Geometry: final body of the model. Coordinates: model frame, mm. A direction names the side the tool comes from. Coordinates: 2 decimals unless noted, no trailing zeros. Write each loop counter-clockwise with the first axis right and the second up, starting at its lowest first coordinate (ties: lowest second). Pieces come first, ordered by that corner, then holes. Notation, with made-up numbers: M 34.5,27.5 L 38.5,27.5 A23 ccw 38.5,49.5 Z; hole C 35.5,89 d7. An arc over 180 degrees is marked long. Write item = value, one per line. Start each with the question number.
Item 1: Reachability of faces 1 (the flat face through (-2.5, -25, 5)), 2 (the flat face through (15, 21, 5)), 3 (the flat face through (-20, 11.5, 7)), 4 (the flat face through (-9, 8, 1)), 5 (the flat face through (-24.2, -15.4, 3.9)) from +Z, -Z, +X, -X, +Y, -Y: full face, straight path, thin tool, end or side. Return the list, or none.
Item 2: Section A-A on y = 21.5. Output: boundary loops of the cut face in (x, z), plus the area to 3 significant figures.
Item 3: Ray query, L1, parallel to X at y = -5, z = 0.75; L2, parallel to Y at x = 15.5, z = 2.75; L3, parallel to Y at x = -16, z = 6. Return the intervals inside material, ascending. Write a range as [from, to].
Item 4: Section C-C on y = -21.5. Output: boundary loops of the cut face in (x, z).
Item 5: Section D-D on y = -10. Output: boundary loops of the cut face in (x, z).
Item 6: First-contact query: pin 1 Ø0.6 at (y, z) = (-17, 0.5) entering from +X; pin 2 Ø6 at (x, y) = (-5.5, -0.5) entering from +Z; pin 3 Ø4 at (y, z) = (1, 4.5) entering from -X; pin 4 Ø10 at (x, y) = (13.5, -2.5) entering from -Z. Flat tips, straight axial feed; report the tip coordinate or a pass-through.
Item 7: Pull-direction query (Y, two-part tool) for faces 6 (the flat face through (0, -6, 0)), 7 (the flat face through (-14, 11, 1)); classes: +Y half, -Y half, draft (parallel to the pull), parting line (faces both ways), or undercut.
Item 8: Section B-B on x = 10. Output: boundary loops of the cut face in (y, z).
from build123d import *

# Parameters (mm, degrees)
SKETCH1_W                                  = 41
SKETCH1_H                                  = 51
BOSS_EXTRUDE1_DEPTH                        = 8
SHELL1_T                                   = -2
CUT_EXTRUDE1_DEPTH                         = 34.264094757
SKETCH3_W                                  = 10
SKETCH3_H                                  = 5
CUT_EXTRUDE2_DEPTH                         = 7
SKETCH4_W                                  = 2
SKETCH4_H                                  = 14
CUT_EXTRUDE3_DEPTH                         = 7
SKETCH5_W                                  = 3.5
SKETCH5_H                                  = 22
CUT_EXTRUDE4_DEPTH                         = 7
SKETCH6_R                                  = 1.75
BOSS_EXTRUDE2_DEPTH                        = 8
MIRROR1_AT_THE_SECOND_PLANE_COPY_1_SKETC_R = 1.75
MIRROR1_AT_THE_SECOND_PLANE_COPY_1_DEPTH   = 8
SKETCH7_W                                  = 9.5
SKETCH7_H                                  = 5.5
BOSS_EXTRUDE3_DEPTH                        = 3
CHAMFER1_SIZE                              = 3


with BuildPart() as part:
    # Sketch1 → Boss-Extrude1 (new body)
    with BuildSketch(Plane.XY):
        Rectangle(SKETCH1_W, SKETCH1_H)
    extrude(amount=BOSS_EXTRUDE1_DEPTH)

    # Shell1
    shell1_openings = [part.faces().sort_by_distance(p)[0] for p in [
        (0, 0, 8),
    ]]
    offset(amount=SHELL1_T, openings=shell1_openings, kind=Kind.INTERSECTION)

    # Sketch2 → Cut-Extrude1 (cut, through all)
    with BuildSketch(Plane.XY.offset(2)):
        Polygon((-9, 23.5), (9, 23.5), (9, 18), (18.5, 18), (18.5, 11), (9, 11), (9, 5.5), (-9, 5.5), (-9, 11), (-18.5, 11), (-18.5, 18), (-9, 18), align=None)
    extrude(amount=-CUT_EXTRUDE1_DEPTH, mode=Mode.SUBTRACT)

    # Sketch3 → Cut-Extrude2 (cut)
    with BuildSketch(Plane.XZ.offset(25.5)):
        with Locations((-7.5, 5.5)):
            Rectangle(SKETCH3_W, SKETCH3_H)
    extrude(amount=-CUT_EXTRUDE2_DEPTH, mode=Mode.SUBTRACT)

    # Sketch4 → Cut-Extrude3 (cut)
    with BuildSketch(Plane.ZY.offset(20.5)):
        with Locations((7, 4.5)):
            Rectangle(SKETCH4_W, SKETCH4_H)
    extrude(amount=-CUT_EXTRUDE3_DEPTH, mode=Mode.SUBTRACT)

    # Sketch5 → Cut-Extrude4 (cut)
    with BuildSketch(Plane(origin=(0, 0, 0), x_dir=(-1, 0, 0), z_dir=(0, 0, -1))):
        with Locations((-16.25, -12.5)):
            Rectangle(SKETCH5_W, SKETCH5_H)
        with Locations((16.25, -12.5)):
            Rectangle(SKETCH5_W, SKETCH5_H)
    extrude(amount=-CUT_EXTRUDE4_DEPTH, mode=Mode.SUBTRACT)

    # Sketch6 → Boss-Extrude2 (add)
    with BuildSketch(Plane.XY):
        with BuildLine():
            Line((25.5, 25.5), (20.5, 25.5))
            Line((20.5, 25.5), (20.5, 12.5))
            Line((20.5, 12.5), (27.967226295, 18.351540947))
            ThreePointArc((27.967226295, 18.351540947), (29.281126566, 22.805021798), (25.5, 25.5))
        make_face()
        with Locations((25.5, 21.5)):
            Circle(SKETCH6_R, mode=Mode.SUBTRACT)
    boss_extrude2 = extrude(amount=BOSS_EXTRUDE2_DEPTH)

    # Mirror1: Boss-Extrude2 across plane
    add(boss_extrude2.mirror(Plane(origin=(0, 0, 0), x_dir=(0, 0, 1), z_dir=(1, 0, 0))))

    # Mirror1 at the second plane: Boss-Extrude2 across plane
    add(boss_extrude2.mirror(Plane.ZX))

    # Mirror1 at the second plane copy 1 sketc → Mirror1 at the second plane copy 1 (add)
    with BuildSketch(Plane(origin=(0, 0, 0), x_dir=(-1, 0, 0), z_dir=(0, 0, 1))):
        with BuildLine():
            Line((25.5, 25.5), (20.5, 25.5))
            Line((20.5, 25.5), (20.5, 12.5))
            Line((20.5, 12.5), (27.967226295, 18.351540947))
            ThreePointArc((27.967226295, 18.351540947), (29.281126566, 22.805021798), (25.5, 25.5))
        make_face()
        with Locations((25.5, 21.5)):
            Circle(MIRROR1_AT_THE_SECOND_PLANE_COPY_1_SKETC_R, mode=Mode.SUBTRACT)
    extrude(amount=MIRROR1_AT_THE_SECOND_PLANE_COPY_1_DEPTH)

    # Sketch7 → Boss-Extrude3 (add)
    with BuildSketch(Plane.XY.offset(2)):
        with Locations((-13.75, 20.75)):
            Rectangle(SKETCH7_W, SKETCH7_H)
        with Locations((13.75, 20.75)):
            Rectangle(SKETCH7_W, SKETCH7_H)
    extrude(amount=BOSS_EXTRUDE3_DEPTH)

    # Chamfer1
    chamfer1_edges = [part.edges().sort_by_distance(p)[0] for p in [
        (-9, 20.75, 5),
        (9, 20.75, 5),
    ]]
    chamfer(chamfer1_edges, length=CHAMFER1_SIZE)


solid = part.part
Responses:
q1.face_1 = +Z, -Y
q1.face_2 = +Z
q1.face_3 = +Z, -X
q1.face_4 = +Z, -Z
q1.face_5 = +Z, -Z, -X
q2.outline = M -29.5,0 L -27.25,0 L -27.25,8 L -29.5,8 Z; M -23.75,0 L -9,0 L -9,2 L -12,5 L -18.5,5 L -18.5,8 L -23.75,8 Z; M 9,0 L 23.75,0 L 23.75,8 L 18.5,8 L 18.5,5 L 12,5 L 9,2 Z; M 27.25,0 L 29.5,0 L 29.5,8 L 27.25,8 Z
q2.area = 206 mm²
q3.L1 = [-20.5, -18], [-14.5, 14.5], [18, 20.5]
q3.L2 = [-25.5, -23.5], [18, 25.5]
q3.L3 = [-25.5, -23.5], [23.5, 25.5]
q4.outline = M -29.5,0 L -27.25,0 L -27.25,8 L -29.5,8 Z; M -23.75,0 L -18,0 L -18,2 L -18.5,2 L -18.5,8 L -23.75,8 Z; M -14.5,0 L 14.5,0 L 14.5,2 L -14.5,2 Z; M 18,0 L 23.75,0 L 23.75,8 L 18.5,8 L 18.5,2 L 18,2 Z; M 27.25,0 L 29.5,0 L 29.5,8 L 27.25,8 Z
q5.outline = M -20.5,0 L -18,0 L -18,2 L -18.5,2 L -18.5,8 L -20.5,8 Z; M -14.5,0 L 14.5,0 L 14.5,2 L -14.5,2 Z; M 18,0 L 20.5,0 L 20.5,8 L 18.5,8 L 18.5,2 L 18,2 Z
q6.pin_1 = 26.63
q6.pin_2 = 2
q6.pin_3 = -20.5
q6.pin_4 = 0
q7.face_6 = draft
q7.face_7 = undercut
q8.outline = M -25.5,0 L 11,0 L 11,2 L -23.5,2 L -23.5,8 L -25.5,8 Z; M 18,0 L 25.5,0 L 25.5,8 L 23.5,8 L 23.5,3 L 18,3 Z
